```python
from build123d import *

# Parameters (mm, degrees)
SKETCH1_R           = 1.45
SKETCH1_W           = 23
SKETCH1_H           = 66
BOSS_EXTRUDE1_DEPTH = 5.85
FILLET1_R           = 4.5
FILLET2_R           = 0.749
FILLET3_R           = 2.5
FILLET4_R           = 2.5


with BuildPart() as part:
    # Sketch1 → Boss-Extrude1 (new body)
    # profile 1 of 4: a face of its own
    with BuildSketch(Plane(origin=(0, 0, 0), x_dir=(1, 0, 0), z_dir=(0, 1, 0))):
        with BuildLine():
            Line((-31.5, 41.25), (-7.2, 41.25))
            ThreePointArc((-7.2, 41.25), (-5.255456352, 42.055456352), (-4.45, 44))
            ThreePointArc((-4.45, 44), (0, 48.45), (4.45, 44))
            ThreePointArc((4.45, 44), (5.255456352, 42.055456352), (7.2, 41.25))
            Line((7.2, 41.25), (31.5, 41.25))
            ThreePointArc((31.5, 41.25), (34.681980515, 39.931980515), (36, 36.75))
            Line((36, 36.75), (36, 18.45))
            ThreePointArc((36, 18.45), (40.100505063, 8.550505063), (50, 4.45))
            ThreePointArc((50, 4.45), (54.45, 0), (50, -4.45))
            ThreePointArc((50, -4.45), (40.100505063, -8.550505063), (36, -18.45))
            Line((36, -18.45), (36, -36.75))
            ThreePointArc((36, -36.75), (34.681980515, -39.931980515), (31.5, -41.25))
            Line((31.5, -41.25), (7.2, -41.25))
            ThreePointArc((7.2, -41.25), (5.255456352, -42.055456352), (4.45, -44))
            ThreePointArc((4.45, -44), (0, -48.45), (-4.45, -44))
            ThreePointArc((-4.45, -44), (-5.255456352, -42.055456352), (-7.2, -41.25))
            Line((-7.2, -41.25), (-31.5, -41.25))
            ThreePointArc((-31.5, -41.25), (-34.681980515, -39.931980515), (-36, -36.75))
            Line((-36, -36.75), (-36, -18.45))
            ThreePointArc((-36, -18.45), (-40.100505063, -8.550505063), (-50, -4.45))
            ThreePointArc((-50, -4.45), (-54.45, 0), (-50, 4.45))
            ThreePointArc((-50, 4.45), (-40.100505063, 8.550505063), (-36, 18.45))
            Line((-36, 18.45), (-36, 36.75))
            ThreePointArc((-36, 36.75), (-34.681980515, 39.931980515), (-31.5, 41.25))
        make_face()
        with Locations(Location((0, 44, 0), (0, 0, 270))):
            Circle(SKETCH1_R, mode=Mode.SUBTRACT)
        with Locations(Location((0, -44, 0), (0, 0, 270))):
            Circle(SKETCH1_R, mode=Mode.SUBTRACT)
        with Locations(Location((-50, 0, 0), (0, 0, 270))):
            Circle(SKETCH1_R, mode=Mode.SUBTRACT)
        with Locations(Location((50, 0, 0), (0, 0, 270))):
            Circle(SKETCH1_R, mode=Mode.SUBTRACT)
        Polygon((31.5, 36.5), (20.5, 36.5), (-31.5, 36.5), (-31.5, -36.5), (20.5, -36.5), (31.5, -36.5), align=None, mode=Mode.SUBTRACT)
    # profile 2 of 4: a face of its own
    with BuildSketch(Plane(origin=(0, 0, 0), x_dir=(1, 0, 0), z_dir=(0, 1, 0))):
        Polygon((-15, 21.090403907), (-15, 23.590403907), (-19, 23.590403907), (-19, 0), (-19, -23.590403907), (-15, -23.590403907), (-15, -21.090403907), (-16.5, -21.090403907), (-16.5, 0), (-16.5, 21.090403907), align=None)
    # profile 3 of 4: a face of its own
    with BuildSketch(Plane(origin=(0, 0, 0), x_dir=(1, 0, 0), z_dir=(0, 1, 0))):
        Polygon((19, 23.590403907), (15, 23.590403907), (15, 21.090403907), (16.5, 21.090403907), (16.5, 0), (16.5, -21.090403907), (15, -21.090403907), (15, -23.590403907), (19, -23.590403907), (19, 0), align=None)
    # profile 4 of 4: a face of its own
    with BuildSketch(Plane(origin=(0, 0, 0), x_dir=(1, 0, 0), z_dir=(0, 1, 0))):
        Polygon((15, 36.5), (-15, 36.5), (-15, 23.590403907), (-15, 21.090403907), (-15, -21.090403907), (-15, -23.590403907), (-15, -36.5), (15, -36.5), (15, -23.590403907), (15, -21.090403907), (15, 21.090403907), (15, 23.590403907), align=None)
        Rectangle(SKETCH1_W, SKETCH1_H, mode=Mode.SUBTRACT)
    extrude(amount=BOSS_EXTRUDE1_DEPTH)

    # Fillet1
    fillet1_edges = [part.edges().sort_by_distance(p)[0] for p in [
        (15, 2.925, -36.5),
        (15, 2.925, 36.5),
        (31.5, 2.925, 36.5),
        (31.5, 2.925, -36.5),
        (-31.5, 2.925, -36.5),
        (-31.5, 2.925, 36.5),
        (-15, 2.925, 36.5),
        (-15, 2.925, -36.5),
    ]]
    fillet(fillet1_edges, radius=FILLET1_R)

    # Fillet2
    fillet2_edges = [part.edges().sort_by_distance(p)[0] for p in [
        (-16.5, 2.925, -21.090403907),
        (-16.5, 2.925, 21.090403907),
        (-15, 2.925, 21.090403907),
        (-15, 2.925, -21.090403907),
        (15, 2.925, 21.090403907),
        (16.5, 2.925, 21.090403907),
        (16.5, 2.925, -21.090403907),
        (15, 2.925, -21.090403907),
    ]]
    fillet(fillet2_edges, radius=FILLET2_R)

    # Fillet3
    fillet3_edges = [part.edges().sort_by_distance(p)[0] for p in [
        (11.5, 2.925, -33),
        (19, 2.925, -23.590403907),
        (19, 2.925, 23.590403907),
        (-19, 2.925, 23.590403907),
        (-19, 2.925, -23.590403907),
        (-11.5, 2.925, -33),
        (-11.5, 2.925, 33),
        (11.5, 2.925, 33),
    ]]
    fillet(fillet3_edges, radius=FILLET3_R)

    # Fillet4
    fillet4_edges = [part.edges().sort_by_distance(p)[0] for p in [
        (15, 2.925, -23.590403907),
        (-15, 2.925, -23.590403907),
        (15, 2.925, 23.590403907),
        (-15, 2.925, 23.590403907),
    ]]
    fillet(fillet4_edges, radius=FILLET4_R)


solid = part.part
```
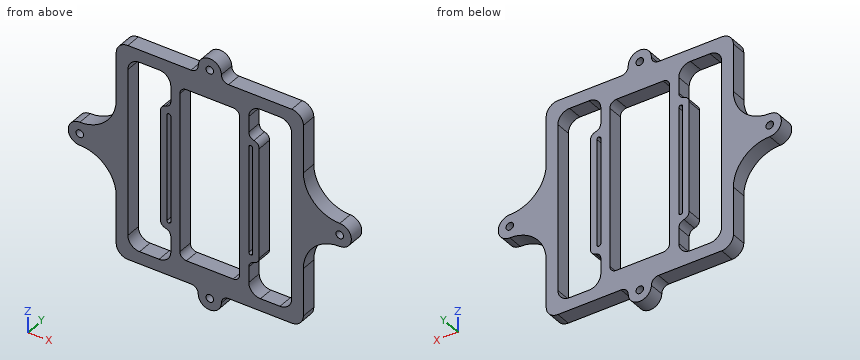
Here's how the part is built. I have some questions about the finished solid (model axes, mm). Give positions to 0.01 mm unless a question says otherwise; leave off trailing zeros. Order: outer loops, then holes, each group sorted by start corner. A loop starts at its lowest first (then second) coordinate and runs counter-clockwise, first axis right, second up. Notation, with made-up numbers: (71, 24) - (85, 24) arc R9 cw to (85, 41) - close; hole circle Ø3 at (49, 30.25). An arc over 180 degrees is marked (long way). Answer as a JSON object with one key per item and string values. Group by question number.
Item 1: Please list where these lines run through material, in increasing order: probe 1 along X at (y, z) = (2.35, -20.5); probe 2 along X at (y, z) = (2.25, -30.5); probe 3 along X at (y, z) = (3, 44).
Item 2: For P1, Ø1.8, axis at y = 3, z = 30, coming from the +X side; P2, Ø1, axis at x = 29, y = 4, coming from the -Z side; P3, Ø12, axis at x = 24, z = 28, coming from the +Y side; P4, Ø3, axis at x = 18.5, y = 3.5, coming from the +Z side, each with a flat end and sliding along its axis, tell me the tip position at first contact or that it passes through.
Item 3: If we section it at C-C on z = 0: Give the number of separate pieces and of enclosed holes in the cut face, and give its area (3 significant figures).
Item 4: If we section it at B-B on x = 0: Please give me the cut outline in (y, z), and give its area (3 significant figures).
Item 5: If we section it at A-A on z = -29: Please give me the cut outline in (x, y), and give its area (3 significant figures).
Result set:
{
 "1": {"probe 1": "-36 to -31.5, -19 to -16.48, -15.02 to -11.5, 11.5 to 15.02, 16.48 to 19, 31.5 to 36", "probe 2": "-36 to -31.5, -15 to -11.5, 11.5 to 15, 31.5 to 36", "probe 3": "-4.45 to -1.45, 1.45 to 4.45"},
 "2": {"P1": "x = 36", "P2": "z = -41.25", "P3": "through", "P4": "z = 41.25"},
 "3": {"separate pieces": "8", "enclosed holes": "0", "area": "305 mm²"},
 "4": {"outline": "(0, -48.45) - (5.85, -48.45) - (5.85, -45.45) - (0, -45.45) - close; (0, -42.55) - (5.85, -42.55) - (5.85, -33) - (0, -33) - close; (0, 33) - (5.85, 33) - (5.85, 42.55) - (0, 42.55) - close; (0, 45.45) - (5.85, 45.45) - (5.85, 48.45) - (0, 48.45) - close", "area": "147 mm²"},
 "5": {"outline": "(-36, 0) - (-31.5, 0) - (-31.5, 5.85) - (-36, 5.85) - close; (-15, 0) - (-11.5, 0) - (-11.5, 5.85) - (-15, 5.85) - close; (11.5, 0) - (15, 0) - (15, 5.85) - (11.5, 5.85) - close; (31.5, 0) - (36, 0) - (36, 5.85) - (31.5, 5.85) - close", "area": "93.6 mm²"}
}
